```python
from build123d import *

# Parameters (mm, degrees)
SKETCH1_W           = 170.9
SKETCH1_H           = 70
BOSS_EXTRUDE1_DEPTH = 5.9
CUT_EXTRUDE1_DEPTH  = 6.9
SKETCH3_W           = 5.9
SKETCH3_H           = 10
CUT_EXTRUDE2_DEPTH  = 6.9
SKETCH4_W           = 5.9
SKETCH4_H           = 10
CUT_EXTRUDE3_DEPTH  = 6.9
CUT_EXTRUDE4_REACH  = 7.9
SKETCH5_R           = 2.05


with BuildPart() as part:
    # Sketch1 → Boss-Extrude1 (new body)
    with BuildSketch(Plane.XY):
        Rectangle(SKETCH1_W, SKETCH1_H)
    extrude(amount=BOSS_EXTRUDE1_DEPTH)

    # Sketch2 → Cut-Extrude1 (cut, through all)
    with BuildSketch(Plane.XY.offset(5.9)):
        Polygon((-50, -21), (-85.45, -21), (-85.45, -35), (85.45, -35), (85.45, -21), (50, -21), (50, -26.9), (57, -26.9), (57, -32), (33, -32), (33, -26.9), (40, -26.9), (40, -21), (5, -21), (5, -26.9), (12, -26.9), (12, -32), (-12, -32), (-12, -26.9), (-5, -26.9), (-5, -21), (-40, -21), (-40, -26.9), (-33, -26.9), (-33, -32), (-57, -32), (-57, -26.9), (-50, -26.9), align=None)
    extrude(amount=-CUT_EXTRUDE1_DEPTH, mode=Mode.SUBTRACT)

    # Sketch3 → Cut-Extrude2 (cut, through all)
    with BuildSketch(Plane.XY.offset(5.9)):
        with Locations((82.5, 20)):
            Rectangle(SKETCH3_W, SKETCH3_H)
        with Locations((82.5, 0)):
            Rectangle(SKETCH3_W, SKETCH3_H)
        with Locations((-82.5, 0)):
            Rectangle(SKETCH3_W, SKETCH3_H)
        with Locations((-82.5, 20)):
            Rectangle(SKETCH3_W, SKETCH3_H)
    extrude(amount=-CUT_EXTRUDE2_DEPTH, mode=Mode.SUBTRACT)

    # Sketch4 → Cut-Extrude3 (cut, through all)
    with BuildSketch(Plane.XY.offset(5.9)):
        with Locations((82.5, 30)):
            Rectangle(SKETCH4_W, SKETCH4_H)
        with Locations((-82.5, 30)):
            Rectangle(SKETCH4_W, SKETCH4_H)
    extrude(amount=-CUT_EXTRUDE3_DEPTH, mode=Mode.SUBTRACT)

    # Sketch5 → Cut-Extrude4 (cut, up to next)
    with BuildSketch(Plane.XY.offset(5.9), mode=Mode.PRIVATE) as cut_extrude4_sk1:
        with Locations((-50, -26.9)):
            Circle(SKETCH5_R)
    cut_extrude4_tool1 = extrude(cut_extrude4_sk1.sketch, amount=-CUT_EXTRUDE4_REACH, mode=Mode.PRIVATE) & part.part
    add(cut_extrude4_tool1.solids().sort_by_distance((-50, -26.9, 5.9))[0], mode=Mode.SUBTRACT)
    # Sketch5 → Cut-Extrude4 (cut, up to next)
    with BuildSketch(Plane.XY.offset(5.9), mode=Mode.PRIVATE) as cut_extrude4_sk2:
        with Locations((-40, -26.9)):
            Circle(SKETCH5_R)
    cut_extrude4_tool2 = extrude(cut_extrude4_sk2.sketch, amount=-CUT_EXTRUDE4_REACH, mode=Mode.PRIVATE) & part.part
    add(cut_extrude4_tool2.solids().sort_by_distance((-40, -26.9, 5.9))[0], mode=Mode.SUBTRACT)
    # Sketch5 → Cut-Extrude4 (cut, up to next)
    with BuildSketch(Plane.XY.offset(5.9), mode=Mode.PRIVATE) as cut_extrude4_sk3:
        with Locations((-50, -21)):
            Circle(SKETCH5_R)
    cut_extrude4_tool3 = extrude(cut_extrude4_sk3.sketch, amount=-CUT_EXTRUDE4_REACH, mode=Mode.PRIVATE) & part.part
    add(cut_extrude4_tool3.solids().sort_by_distance((-50, -21, 5.9))[0], mode=Mode.SUBTRACT)
    # Sketch5 → Cut-Extrude4 (cut, up to next)
    with BuildSketch(Plane.XY.offset(5.9), mode=Mode.PRIVATE) as cut_extrude4_sk4:
        with Locations((-40, -21)):
            Circle(SKETCH5_R)
    cut_extrude4_tool4 = extrude(cut_extrude4_sk4.sketch, amount=-CUT_EXTRUDE4_REACH, mode=Mode.PRIVATE) & part.part
    add(cut_extrude4_tool4.solids().sort_by_distance((-40, -21, 5.9))[0], mode=Mode.SUBTRACT)
    # Sketch5 → Cut-Extrude4 (cut, up to next)
    with BuildSketch(Plane.XY.offset(5.9), mode=Mode.PRIVATE) as cut_extrude4_sk5:
        with Locations((-5, -21)):
            Circle(SKETCH5_R)
    cut_extrude4_tool5 = extrude(cut_extrude4_sk5.sketch, amount=-CUT_EXTRUDE4_REACH, mode=Mode.PRIVATE) & part.part
    add(cut_extrude4_tool5.solids().sort_by_distance((-5, -21, 5.9))[0], mode=Mode.SUBTRACT)
    # Sketch5 → Cut-Extrude4 (cut, up to next)
    with BuildSketch(Plane.XY.offset(5.9), mode=Mode.PRIVATE) as cut_extrude4_sk6:
        with Locations((5, -21)):
            Circle(SKETCH5_R)
    cut_extrude4_tool6 = extrude(cut_extrude4_sk6.sketch, amount=-CUT_EXTRUDE4_REACH, mode=Mode.PRIVATE) & part.part
    add(cut_extrude4_tool6.solids().sort_by_distance((5, -21, 5.9))[0], mode=Mode.SUBTRACT)
    # Sketch5 → Cut-Extrude4 (cut, up to next)
    with BuildSketch(Plane.XY.offset(5.9), mode=Mode.PRIVATE) as cut_extrude4_sk7:
        with Locations((-5, -26.9)):
            Circle(SKETCH5_R)
    cut_extrude4_tool7 = extrude(cut_extrude4_sk7.sketch, amount=-CUT_EXTRUDE4_REACH, mode=Mode.PRIVATE) & part.part
    add(cut_extrude4_tool7.solids().sort_by_distance((-5, -26.9, 5.9))[0], mode=Mode.SUBTRACT)
    # Sketch5 → Cut-Extrude4 (cut, up to next)
    with BuildSketch(Plane.XY.offset(5.9), mode=Mode.PRIVATE) as cut_extrude4_sk8:
        with Locations((5, -26.9)):
            Circle(SKETCH5_R)
    cut_extrude4_tool8 = extrude(cut_extrude4_sk8.sketch, amount=-CUT_EXTRUDE4_REACH, mode=Mode.PRIVATE) & part.part
    add(cut_extrude4_tool8.solids().sort_by_distance((5, -26.9, 5.9))[0], mode=Mode.SUBTRACT)
    # Sketch5 → Cut-Extrude4 (cut, up to next)
    with BuildSketch(Plane.XY.offset(5.9), mode=Mode.PRIVATE) as cut_extrude4_sk9:
        with Locations((40, -26.9)):
            Circle(SKETCH5_R)
    cut_extrude4_tool9 = extrude(cut_extrude4_sk9.sketch, amount=-CUT_EXTRUDE4_REACH, mode=Mode.PRIVATE) & part.part
    add(cut_extrude4_tool9.solids().sort_by_distance((40, -26.9, 5.9))[0], mode=Mode.SUBTRACT)
    # Sketch5 → Cut-Extrude4 (cut, up to next)
    with BuildSketch(Plane.XY.offset(5.9), mode=Mode.PRIVATE) as cut_extrude4_sk10:
        with Locations((50, -26.9)):
            Circle(SKETCH5_R)
    cut_extrude4_tool10 = extrude(cut_extrude4_sk10.sketch, amount=-CUT_EXTRUDE4_REACH, mode=Mode.PRIVATE) & part.part
    add(cut_extrude4_tool10.solids().sort_by_distance((50, -26.9, 5.9))[0], mode=Mode.SUBTRACT)
    # Sketch5 → Cut-Extrude4 (cut, up to next)
    with BuildSketch(Plane.XY.offset(5.9), mode=Mode.PRIVATE) as cut_extrude4_sk11:
        with Locations((50, -21)):
            Circle(SKETCH5_R)
    cut_extrude4_tool11 = extrude(cut_extrude4_sk11.sketch, amount=-CUT_EXTRUDE4_REACH, mode=Mode.PRIVATE) & part.part
    add(cut_extrude4_tool11.solids().sort_by_distance((50, -21, 5.9))[0], mode=Mode.SUBTRACT)
    # Sketch5 → Cut-Extrude4 (cut, up to next)
    with BuildSketch(Plane.XY.offset(5.9), mode=Mode.PRIVATE) as cut_extrude4_sk12:
        with Locations((40, -21)):
            Circle(SKETCH5_R)
    cut_extrude4_tool12 = extrude(cut_extrude4_sk12.sketch, amount=-CUT_EXTRUDE4_REACH, mode=Mode.PRIVATE) & part.part
    add(cut_extrude4_tool12.solids().sort_by_distance((40, -21, 5.9))[0], mode=Mode.SUBTRACT)
    # Sketch5 → Cut-Extrude4 (cut, up to next)
    with BuildSketch(Plane.XY.offset(5.9), mode=Mode.PRIVATE) as cut_extrude4_sk13:
        with Locations((79.55, -5)):
            Circle(SKETCH5_R)
    cut_extrude4_tool13 = extrude(cut_extrude4_sk13.sketch, amount=-CUT_EXTRUDE4_REACH, mode=Mode.PRIVATE) & part.part
    add(cut_extrude4_tool13.solids().sort_by_distance((79.55, -5, 5.9))[0], mode=Mode.SUBTRACT)
    # Sketch5 → Cut-Extrude4 (cut, up to next)
    with BuildSketch(Plane.XY.offset(5.9), mode=Mode.PRIVATE) as cut_extrude4_sk14:
        with Locations((79.55, 5)):
            Circle(SKETCH5_R)
    cut_extrude4_tool14 = extrude(cut_extrude4_sk14.sketch, amount=-CUT_EXTRUDE4_REACH, mode=Mode.PRIVATE) & part.part
    add(cut_extrude4_tool14.solids().sort_by_distance((79.55, 5, 5.9))[0], mode=Mode.SUBTRACT)
    # Sketch5 → Cut-Extrude4 (cut, up to next)
    with BuildSketch(Plane.XY.offset(5.9), mode=Mode.PRIVATE) as cut_extrude4_sk15:
        with Locations((79.55, 15)):
            Circle(SKETCH5_R)
    cut_extrude4_tool15 = extrude(cut_extrude4_sk15.sketch, amount=-CUT_EXTRUDE4_REACH, mode=Mode.PRIVATE) & part.part
    add(cut_extrude4_tool15.solids().sort_by_distance((79.55, 15, 5.9))[0], mode=Mode.SUBTRACT)
    # Sketch5 → Cut-Extrude4 (cut, up to next)
    with BuildSketch(Plane.XY.offset(5.9), mode=Mode.PRIVATE) as cut_extrude4_sk16:
        with Locations((-79.55, 15)):
            Circle(SKETCH5_R)
    cut_extrude4_tool16 = extrude(cut_extrude4_sk16.sketch, amount=-CUT_EXTRUDE4_REACH, mode=Mode.PRIVATE) & part.part
    add(cut_extrude4_tool16.solids().sort_by_distance((-79.55, 15, 5.9))[0], mode=Mode.SUBTRACT)
    # Sketch5 → Cut-Extrude4 (cut, up to next)
    with BuildSketch(Plane.XY.offset(5.9), mode=Mode.PRIVATE) as cut_extrude4_sk17:
        with Locations((-79.55, 5)):
            Circle(SKETCH5_R)
    cut_extrude4_tool17 = extrude(cut_extrude4_sk17.sketch, amount=-CUT_EXTRUDE4_REACH, mode=Mode.PRIVATE) & part.part
    add(cut_extrude4_tool17.solids().sort_by_distance((-79.55, 5, 5.9))[0], mode=Mode.SUBTRACT)
    # Sketch5 → Cut-Extrude4 (cut, up to next)
    with BuildSketch(Plane.XY.offset(5.9), mode=Mode.PRIVATE) as cut_extrude4_sk18:
        with Locations((-79.55, -5)):
            Circle(SKETCH5_R)
    cut_extrude4_tool18 = extrude(cut_extrude4_sk18.sketch, amount=-CUT_EXTRUDE4_REACH, mode=Mode.PRIVATE) & part.part
    add(cut_extrude4_tool18.solids().sort_by_distance((-79.55, -5, 5.9))[0], mode=Mode.SUBTRACT)


solid = part.part
```
Geometry: final body of the model. Coordinates: model frame, mm. A direction names the side the tool comes from. Coordinates: 2 decimals unless noted, no trailing zeros. Order: outer loops, then holes, each group sorted by start corner. A loop starts at its lowest first (then second) coordinate and runs counter-clockwise, first axis right, second up.
Item 1: Material intervals for line 1 along Y through (x, z) = (56.5, 2.3); line 2 along X through (y, z) = (6, 3.4); line 3 along X through (y, z) = (0.5, 3.95), sorted ascending.
Answer:
line 1: y = -32 to -26.9, -21 to 35
line 2: x = -85.45 to -81.34, -77.76 to 77.76, 81.34 to 85.45
line 3: x = -79.55 to 79.55
Item 2: Draft query along Y for faces 6 (the face through (83, 15, 3)), 7 (the face through (48.6, -19.5, 3)), 8 (the face through (-57, -29, 3)). Return one class per face: released by +Y, released by -Y, zero draft, split by the parting line, or undercut.
Answer:
face 6: released by +Y
face 7: undercut
face 8: zero draft
Item 3: Section query A-A (x = -61). Output: boundary loops of the cut face in (y, z).
Answer:
outline: (-21, 0) - (35, 0) - (35, 5.9) - (-21, 5.9) - close
Item 4: Access query for faces 1 (the face through (-1, 2, 0)), 2 (the face through (23, -21, 3)), 3 (the face through (0, -32, 3)), 4 (the face through (12, -29, 3)), 5 (the face through (54, -26.9, 3)). Directions: +Z, -Z, +X, -X, +Y, -Y. A direction counts if a zero-diameter tool reaches every point of the face in a straight line with its end or side. Return the directions, or none.
Answer:
face 1: -Z, +X, -X, +Y, -Y
face 2: +Z, -Z
face 3: +Z, -Z, +X, -X, -Y
face 4: +Z, -Z, -Y
face 5: +Z, -Z, +X
Item 5: Section query B-B (y = 20). Output: boundary loops of the cut face in (x, z).
Answer:
outline: (-79.55, 0) - (79.55, 0) - (79.55, 5.9) - (-79.55, 5.9) - close
Item 6: Contact query for flat-ended pins moving along their axis: P1, Ø1.5, axis at y = -24.5, z = 4.5, coming from the -X side; P2, Ø5.5, axis at x = 50, y = -26.9, coming from the +Z side; P3, Ø2.5, axis at y = -28.5, z = 4, coming from the +X side; P4, Ø1.5, axis at y = -22, z = 2.5, coming from the -X side. Output: stop coordinate, or through.
Answer:
P1: stops at x = -50
P2: stops at z = 5.9
P3: stops at x = 57
P4: stops at x = -48.93
